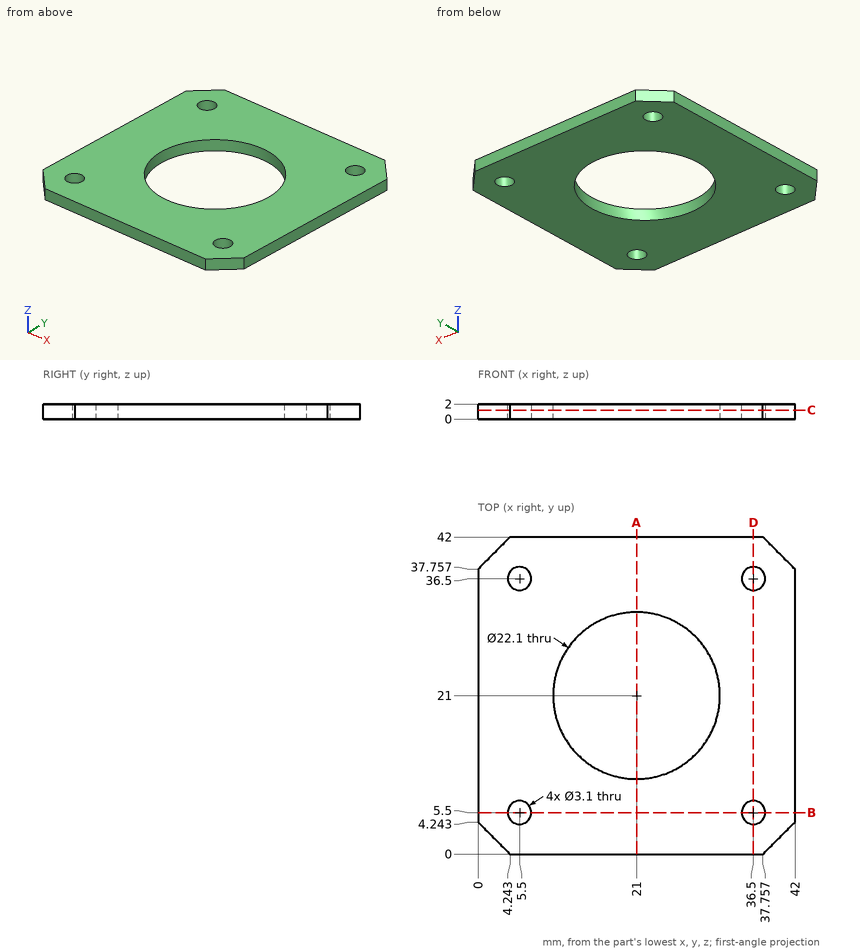
Here's the drawing with two shaded views (mm, measured from the low corner). I have some questions. Give positions to 0.01 mm unless a question says otherwise; leave off trailing zeros. Write each loop counter-clockwise with the first axis right and the second up, starting at its lowest first coordinate (ties: lowest second). Pieces come first, ordered by that corner, then holes. Notation, with made-up numbers: (43, 24) - (75, 24) arc R14 ccw to (75, 49) - close; hole circle Ø10 at (67.5, 6). An arc over 180 degrees is marked (long way). One line per item, written item: value. Start each with the question number.
Item 1: Imagine slicing it at B-B, the plane y = 5.5. List the corners of the cut face in (x, z) for me.
Item 2: Imagine slicing it at A-A, the plane x = 21. List the corners of the cut face in (y, z) for me, and give its area (3 significant figures).
Item 3: Please list where these lines run through material, in increasing order: line 1 (Y direction, x = 5.5, z = 1.4); line 2 (X direction, y = 37, z = 0.35); line 3 (Y direction, x = 21, z = 1.15). Write a range as from..to.
Item 4: Imagine slicing it at C-C, the plane z = 1.2. List the corners of the cut face in (x, y) for me.
Geometry says:
1. outline: (0, 0) - (3.95, 0) - (3.95, 2) - (0, 2) - close; (7.05, 0) - (34.95, 0) - (34.95, 2) - (7.05, 2) - close; (38.05, 0) - (42, 0) - (42, 2) - (38.05, 2) - close
2. outline: (0, 0) - (9.95, 0) - (9.95, 2) - (0, 2) - close; (32.05, 0) - (42, 0) - (42, 2) - (32.05, 2) - close
2. area: 39.8 mm^2
3. line 1: 0..3.95, 7.05..34.95, 38.05..42
3. line 2: 0..4.03, 6.97..35.03, 37.97..42
3. line 3: 0..9.95, 32.05..42
4. outline: (0, 4.24) - (4.24, 0) - (37.76, 0) - (42, 4.24) - (42, 37.76) - (37.76, 42) - (4.24, 42) - (0, 37.76) - close; hole circle Ø3.1 at (5.5, 5.5); hole circle Ø3.1 at (5.5, 36.5); hole circle Ø22.1 at (21, 21); hole circle Ø3.1 at (36.5, 5.5); hole circle Ø3.1 at (36.5, 36.5)
